Read the model definition and answer for the solid it produces. Units are mm, in the model's axes. Face numbers are marked on the shaded views. A direction names the side the tool comes from. Coordinates: 2 decimals unless noted, no trailing zeros. Write each loop counter-clockwise with the first axis right and the second up, starting at its lowest first coordinate (ties: lowest second). Pieces come first, ordered by that corner, then holes. Notation, with made-up numbers: (45.5, 85) -> (84.5, 85) arc R19 cw to (84.5, 108) -> close; hole circle Ø11 at (-35, 37). An arc over 180 degrees is marked (long way). Return JSON: item names as keys, results as strings.
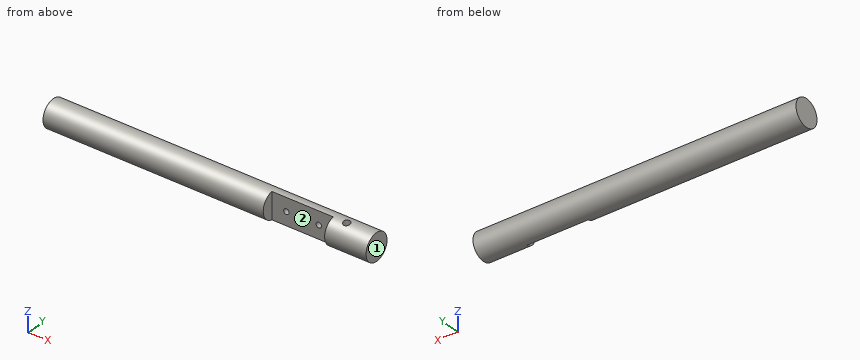
from build123d import *

# Parameters (mm, degrees)
SKETCH1_R                = 1
SKETCH1_R_2              = 0.5
BOSS_EXTRUDE1_DEPTH      = 1.5
SKETCH2_W                = 5.75
SKETCH2_H                = 4
CUT_EXTRUDE1_DEPTH       = 1
BOSS_EXTRUDE2_DEPTH      = 25
BOSS_EXTRUDE2_DEPTH_BACK = 125
BOSS_EXTRUDE2_START      = 8.5
SKETCH5_R                = 6.25
SKETCH6_W                = 28.5
SKETCH6_H                = 12.5
CUT_EXTRUDE2_DEPTH       = 25
SKETCH7_R                = 1.25
CUT_EXTRUDE3_DEPTH       = 3.175
CUT_EXTRUDE4_REACH       = 119.335
CUT_EXTRUDE4_END_RADIUS  = 6.25
SKETCH8_R                = 1.5875


with BuildPart() as part:
    # Sketch1 → Boss-Extrude1 (new, symmetric)
    with BuildSketch(Plane.XY):
        Polygon((-8.5, -19.85), (-8.5, 0), (8.5, 0), (8.5, -19.85), (14.25, -19.85), (14.25, 10), (-14.25, 10), (-14.25, -19.85), align=None)
        with Locations((-7.5, 5)):
            Circle(SKETCH1_R, mode=Mode.SUBTRACT)
        with Locations((7.5, 5)):
            Circle(SKETCH1_R, mode=Mode.SUBTRACT)
        with Locations((-11.375, -17.35)):
            Circle(SKETCH1_R_2, mode=Mode.SUBTRACT)
        with Locations((11.375, -17.35)):
            Circle(SKETCH1_R_2, mode=Mode.SUBTRACT)
    extrude(amount=BOSS_EXTRUDE1_DEPTH, both=True)

    # Sketch2 → Cut-Extrude1 (cut)
    with BuildSketch(Plane.XY.offset(1.5)):
        with Locations((-11.375, -17.85)):
            Rectangle(SKETCH2_W, SKETCH2_H)
        with Locations((11.375, -17.85)):
            Rectangle(SKETCH2_W, SKETCH2_H)
    extrude(amount=-CUT_EXTRUDE1_DEPTH, mode=Mode.SUBTRACT)

    # Sketch5 → Boss-Extrude2 (add, two sides: drawn at the far end of the back side and taken through both)
    with BuildSketch(Plane(origin=(0, 0, 0), x_dir=(0, 0, -1), z_dir=(1, 0, 0)).offset(BOSS_EXTRUDE2_START - BOSS_EXTRUDE2_DEPTH_BACK)):
        with Locations(Location((0, 6.25, 0), (0, 0, 270))):
            Circle(SKETCH5_R)
    extrude(amount=BOSS_EXTRUDE2_DEPTH + BOSS_EXTRUDE2_DEPTH_BACK)

    # Sketch6 → Cut-Extrude2 (cut)
    with BuildSketch(Plane.XZ.offset(19.85)):
        Rectangle(SKETCH6_W, SKETCH6_H)
    extrude(amount=-CUT_EXTRUDE2_DEPTH, mode=Mode.SUBTRACT)

    # Sketch7 → Cut-Extrude3 (cut)
    with BuildSketch(Plane(origin=(0, 5.15, 0), x_dir=(-1, 0, 0), z_dir=(0, -1, 0))):
        with Locations(Location((7.5, 0, 0), (0, 0, 180))):
            Circle(SKETCH7_R)
        with Locations(Location((-7.5, 0, 0), (0, 0, 180))):
            Circle(SKETCH7_R)
    extrude(amount=-CUT_EXTRUDE3_DEPTH, mode=Mode.SUBTRACT)

    # Cut-Extrude4: up to this cylinder (the profile starts inside it)
    cut_extrude4_end = Plane(origin=(20.6, 6.25, 0), z_dir=(-1, 0, 0)) * Cylinder(CUT_EXTRUDE4_END_RADIUS, 252.17, mode=Mode.PRIVATE)
    # Sketch8 → Cut-Extrude4 (cut, up to the surface)
    with BuildSketch(Plane.XY, mode=Mode.PRIVATE) as cut_extrude4_sk1:
        with Locations(Location((20.6, 5.15, 0), (0, 0, 180))):
            Circle(SKETCH8_R)
    cut_extrude4_tool1 = extrude(cut_extrude4_sk1.sketch, amount=CUT_EXTRUDE4_REACH, mode=Mode.PRIVATE) & cut_extrude4_end
    add(cut_extrude4_tool1.solids().sort_by_distance((20.6, 5.15, 0))[0], mode=Mode.SUBTRACT)


solid = part.part
1. The part is cut by section A-A (z = -3.75). Determine the outline of the cut face in (x, y).
Taken from the geometry:
{"outline": "(-116.5, 1.25) -> (-14.25, 1.25) -> (-14.25, 5.15) -> (14.25, 5.15) -> (14.25, 1.25) -> (33.5, 1.25) -> (33.5, 11.25) -> (-116.5, 11.25) -> close"}
2. The part is cut by section D-D (x = 7.5). Determine the outline of the cut face in (y, z) (3 decimals), then the cut area to 3 significant figures.
Taken from the geometry:
{"outline": "(5.15, -6.152) arc R6.25 ccw (long way) to (5.15, 6.152) -> (5.15, 1.25) -> (8.325, 1.25) -> (8.325, -1.25) -> (5.15, -1.25) -> close", "area": "67.1 mm2"}
3. Consider L1, parallel to Z at x = 7.5, y = 7.35; L2, parallel to X at y = 4.25, z = -1.25; L3, parallel to Z at x = -90.5, y = 7.5. Determine where each line is inside the solid, lowest interval first.
Taken from the geometry:
{"L1": "z = -6.15 to -1.25, 1.25 to 6.15", "L2": "x = -116.5 to -14.25, 14.25 to 33.5", "L3": "z = -6.12 to 6.12"}
4. The part is cut by section B-B (x = -28). Determine the outline of the cut face in (y, z).
Taken from the geometry:
{"outline": "circle Ø12.5 at (6.25, 0)"}
5. A tool of negligible diameter and unlimited length cuts with its end or side. For the marked faces 1 and 2, from which of +Z, -Z, +X, -X, +Y, -Y can it reach the whole face along a straight path? Write none if from no direction.
Taken from the geometry:
{"face 1": "+Z, -Z, +X, +Y, -Y", "face 2": "+Z, -Z, -Y"}
6. Flat-ended cylindrical pins translate along their axes: pin 1 Ø3.5 at (x, z) = (0, 1.5) entering from -Y; pin 2 Ø1 at (x, z) = (-71.5, 0.5) entering from -Y; pin 3 Ø2 at (x, z) = (7, 0) entering from -Y. Find the tip coordinate at first contact, or state that the pin passes through.
Taken from the geometry:
{"pin 1": "stops at y = 5.15", "pin 2": "stops at y = 0", "pin 3": "stops at y = 5.15"}
7. The part is cut by section C-C (y = 11.25). Determine the outline of the cut face in (x, z).
Taken from the geometry:
{"outline": "(-116.5, -3.75) -> (33.5, -3.75) -> (33.5, 3.75) -> (-116.5, 3.75) -> close"}
